Part model, mm, in its own coordinate system. A direction names the side the tool comes from. Coordinates: 2 decimals unless noted, no trailing zeros. Order: outer loops, then holes, each group sorted by start corner. A loop starts at its lowest first (then second) coordinate and runs counter-clockwise, first axis right, second up. Notation, with made-up numbers: (-0.5, 43.25) - (22.5, 43.25) arc R14 cw to (22.5, 49.25) - close; hole circle Ø10 at (-15, 33). An arc over 180 degrees is marked (long way). Use a Markdown table: item, result. Add a question column.
1) Saw through at A-A on x = 40. List the corners of the cut face in (y, z), then the cut area to 3 significant figures.
2) Drop flat-ended pins along their axis: P1, Ø9.5, axis at x = 11, z = 19.5, coming from the -Y side; P2, Ø1, axis at y = 27, z = 27, coming from the +X side; P3, Ø14.5, axis at y = 6, z = 24.5, coming from the -X side. Give the stop position or say it passes through.
3) Wall check: L1, parallel to Z at x = 16, y = 16.5; L2, parallel to X at y = 14, z = 19; L3, parallel to Y at x = 39.5, z = 18. Give the ranges that are in metal, low to high. Write a range as [from, to].
4) Saw through at B-B on z = 20.5. List the corners of the cut face in (x, y), then the cut area to 3 significant figures.
5) Tool access for faces 1 (the face through (44.36, 24.99, 22.36)), 2 (the face through (39, 18.416, 20)), 3 (the face through (9, 9, 12.7)): list every direction of +Z, -Z, +X, -X, +Y, -Y with a clear straight run to the whole face (end or side of a thin tool).
6) Saw through at D-D on x = 26. List the corners of the cut face in (y, z), then the cut area to 3 significant figures.
7) Saw through at C-C on y = 8. List the corners of the cut face in (x, z), then the cut area to 3 significant figures.
```python
from build123d import *

# Parameters (mm, degrees)
F0_W      = 50.8
F0_H      = 31.75
F1_DEPTH  = 12.7
F2_W      = 50.8
F2_H      = 13.333772
F3_DEPTH  = 19.05
F5_DEPTH  = 25.4
F7_W      = 12.7
F7_H      = 19.05
F8_DEPTH  = 19.05
F10_DEPTH = 19.05


with BuildPart() as f1:
    # F0 (on Top) → F1 (new body)
    with BuildSketch(Plane.XY):
        with Locations((25.4, 15.875)):
            Rectangle(F0_W, F0_H)
    extrude(amount=F1_DEPTH)

    # F2 (on face) → F3 (join)
    with BuildSketch(Plane.XY.offset(12.7)):
        with Locations((25.4, 25.083114)):
            Rectangle(F2_W, F2_H)
    extrude(amount=F3_DEPTH)

    # F4 (on face) → F5 (cut)
    with BuildSketch(Plane.XZ.offset(-18.416228)):
        Polygon((38.1, 31.75), (50.8, 12.7), (50.8, 31.75), align=None)
    extrude(amount=-F5_DEPTH, mode=Mode.SUBTRACT)

    # F7 (on face) → F8 (join)
    with BuildSketch(Plane.XY.offset(12.7)):
        with Locations((25.4, 9.525)):
            Rectangle(F7_W, F7_H)
    extrude(amount=F8_DEPTH)

    # F9 (on face) → F10 (cut)
    with BuildSketch(Plane.YZ.offset(31.75)):
        Polygon((0, 12.7), (18.416228, 31.75), (0, 31.75), align=None)
    extrude(amount=-F10_DEPTH, mode=Mode.SUBTRACT)


solid = f1.part
```
Results are:
| question | item | result |
|---|---|---|
| 1 | outline | (0, 0) - (31.75, 0) - (31.75, 28.9) - (18.42, 28.9) - (18.42, 12.7) - (0, 12.7) - close |
| 1 | area | 619 mm2 |
| 2 | P1 | y = 18.42 |
| 2 | P2 | x = 41.6 |
| 2 | P3 | x = 19.05 |
| 3 | L1 | [0, 12.7] |
| 3 | L2 | [19.05, 31.75] |
| 3 | L3 | [18.42, 31.75] |
| 4 | outline | (0, 18.42) - (19.05, 18.42) - (19.05, 7.54) - (31.75, 7.54) - (31.75, 18.42) - (45.6, 18.42) - (45.6, 31.75) - (0, 31.75) - close |
| 4 | area | 746 mm2 |
| 5 | face 1 | +Z, +X, +Y, -Y |
| 5 | face 2 | +Z, +X, -Y |
| 5 | face 3 | +Z, -X, -Y |
| 6 | outline | (0, 0) - (31.75, 0) - (31.75, 31.75) - (18.42, 31.75) - (0, 12.7) - close |
| 6 | area | 833 mm2 |
| 7 | outline | (0, 0) - (50.8, 0) - (50.8, 12.7) - (31.75, 12.7) - (31.75, 20.98) - (19.05, 20.98) - (19.05, 12.7) - (0, 12.7) - close |
| 7 | area | 750 mm2 |
